Source: CAD feature listing. Evaluate the final solid. Frame: model axes, mm. A direction names the side the tool comes from. Coordinates: 2 decimals unless noted, no trailing zeros. Write each loop counter-clockwise with the first axis right and the second up, starting at its lowest first coordinate (ties: lowest second). Pieces come first, ordered by that corner, then holes. Notation, with made-up numbers: M 14,42 L 67,42 A13 ccw 67,52 Z; hole C 78.25,65 d4. An arc over 180 degrees is marked long. One line per item, written item: value. Start each with the question number.
Item 1: Mould query, pull axis X, two halves, no side actions, for faces 4 (the cylindrical face through (-35.623, 22.327, 5.848)), 5 (the cylindrical face through (35.147, 5.151, -36.085)), 6 (the flat face through (-13, 10.16, -20)). Classes: released by +X, released by -X, zero draft, split by the parting line, or undercut.
Item 2: Set-up query: faces 1 (the flat face through (-12.646, 22, 6)), 2 (the cylindrical face through (-60.439, 5.151, -36.085)), 3 (the flat face through (-32, 23, 0)). Return all of +Z, -Z, +X, -X, +Y, -Y with unobstructed straight access to the full face (end or side cutting, diameter ignored); none if empty.
Item 3: Ray query, L1, parallel to Z at x = -47, y = 18; L2, parallel to Y at x = -59, z = -36; L3, parallel to X at y = 22, z = 1. Return the intervals inside material, ascending. Write a range as from..to.
Item 4: Cut plane B-B, the plane x = -37.5. Output: boundary loops of the cut face in (y, z).
Item 5: Cut plane C-C, the plane z = -6.5. Output: boundary loops of the cut face in (x, y).
Item 6: Cut plane A-A, the plane y = 36.5. Output: boundary loops of the cut face in (x, z), then the cut area to 3 significant figures.
Item 7: Pin query (flat end, axial travel): P1, Ø15, axis at x = -8, z = -13.5, coming from the +Y side; P2, Ø18, axis at x = -38.05, y = 33.24, coming from the -Z side; P3, Ø13.5, axis at x = -30.5, y = 42, coming from the -Z side; P4, Ø13, axis at y = 17.5, z = 6.5, coming from the +X side. Return the tip coordinate at first contact, or that it passes through.
Item 8: Cut plane D-D, the plane x = -25. Output: boundary loops of the cut face in (y, z), then the cut area to 3 significant figures.
```python
from build123d import *

# Parameters (mm, degrees)
BOSS_EXTRUDE1_DEPTH = 10.16
SKETCH3_W           = 50.8
SKETCH3_H           = 24.064486013
BOSS_EXTRUDE2_DEPTH = 11.8629
SKETCH4_R           = 11.176966962
CUT_EXTRUDE2_DEPTH  = 12.862900188
FILLET1_R           = 10
FILLET2_R           = 10
FILLET3_R           = 10


with BuildPart() as part:
    # Sketch1 → Boss-Extrude1 (new body)
    with BuildSketch(Plane(origin=(0, 0, 0), x_dir=(1, 0, 0), z_dir=(0, 1, 0))):
        Polygon((38.154070096, 38.937099812), (-63.445929904, 38.937099812), (-63.445929904, -11.862900188), (-12.645929904, -11.862900188), (38.154070096, 21.8411914), align=None)
    extrude(amount=BOSS_EXTRUDE1_DEPTH)

    # Sketch3 → Boss-Extrude2 (add)
    with BuildSketch(Plane.XY):
        with BuildLine():
            ThreePointArc((-63.445929904, 34.224486013), (-38.045929904, 54.474648718), (-12.645929904, 34.224486013))
            Line((-12.645929904, 34.224486013), (-63.445929904, 34.224486013))
        make_face()
        with Locations((-38.045929904, 22.192243007)):
            Rectangle(SKETCH3_W, SKETCH3_H)
    extrude(amount=BOSS_EXTRUDE2_DEPTH)

    # Sketch4 → Cut-Extrude2 (cut, through all)
    with BuildSketch(Plane(origin=(0, 0, 0), x_dir=(-1, 0, 0), z_dir=(0, 0, -1))):
        with Locations((38.045929904, 33.23792349)):
            Circle(SKETCH4_R)
    extrude(amount=-CUT_EXTRUDE2_DEPTH, mode=Mode.SUBTRACT)

    # Fillet1
    fillet1_edges = [part.edges().sort_by_distance(p)[0] for p in [
        (38.154070096, 5.08, -38.937099812),
    ]]
    fillet(fillet1_edges, radius=FILLET1_R)

    # Fillet2
    fillet2_edges = [part.edges().sort_by_distance(p)[0] for p in [
        (38.154070096, 5.08, -21.8411914),
    ]]
    fillet(fillet2_edges, radius=FILLET2_R)

    # Fillet3
    fillet3_edges = [part.edges().sort_by_distance(p)[0] for p in [
        (-63.445929904, 5.08, -38.937099812),
    ]]
    fillet(fillet3_edges, radius=FILLET3_R)


solid = part.part
```
From the geometry:
1. face 4: undercut
1. face 5: released by +X
1. face 6: zero draft
2. face 1: +Z, -Z, +X, +Y
2. face 2: -Z, -X, +Y, -Y
2. face 3: -Z, +X, -X, +Y
3. L1: z = 0..11.86
3. L2: y = 0..10.16
3. L3: x = -63.45..-12.65
4. outline: M 0,-38.94 L 10.16,-38.94 L 10.16,0 L 22.07,0 L 22.07,11.86 L 0,11.86 Z; M 44.4,0 L 54.47,0 L 54.47,11.86 L 44.4,11.86 Z
5. outline: M -63.45,0 L 15.03,0 L 15.03,10.16 L -63.45,10.16 Z
6. outline: M -62.82,0 L -48.74,0 L -48.74,11.86 L -62.82,11.86 Z; M -27.36,0 L -13.28,0 L -13.28,11.86 L -27.36,11.86 Z
6. area: 334 mm²
7. P1: stops at y = 10.16
7. P2: passes through
7. P3: stops at z = 0
7. P4: stops at x = -12.65
8. outline: M 0,-38.94 L 10.16,-38.94 L 10.16,0 L 50.97,0 L 50.97,11.86 L 0,11.86 Z
8. area: 1,000 mm²
